Verification items for the finished model (mm, model axes). A direction names the side the tool comes from. Coordinates: 2 decimals unless noted, no trailing zeros. Write each loop counter-clockwise with the first axis right and the second up, starting at its lowest first coordinate (ties: lowest second). Pieces come first, ordered by that corner, then holes. Notation, with made-up numbers: M 79,73 L 110,73 A21 ccw 110,81 Z; hole C 29.5,68.5 d8. An arc over 180 degrees is marked long. Answer in a Markdown table with one row per item.
from build123d import *

# Parameters (mm, degrees)
F1_DEPTH = 88.9


with BuildPart() as f1:
    # F0 (on Front) → F1 (new body)
    with BuildSketch(Plane.XZ):
        Polygon((53.412888, 0), (0, 167.077348), (-5.068147, 167.077348), (-64.475396, 4.895769), (-73.939636, 8.340181), (-71.767969, 14.307288), (-75.421233, 15.636856), (-77.5929, 9.669749), (-79.330342, 4.895769), (-79.330342, 0), (-66.222783, 0.125408), (-61.154637, 0.125408), (-41.877323, 52.752407), (-2.916649, 52.752407), (31.086335, 52.752407), (48.650388, 0), align=None)
        Polygon((29.563813, 57.514907), (-2.916649, 57.514907), (-40.132815, 57.514907), (-2.916649, 159.114907), align=None, mode=Mode.SUBTRACT)
    extrude(amount=F1_DEPTH)


solid = f1.part
1) Thickness scan on L1, parallel to X at y = -52, z = 67; L2, parallel to X at y = -20, z = 153.5; L3, parallel to X at y = -71.5, z = 57. Record the ranges inside material, lowest first. Write a range as [from, to].
Response values:
| item | result |
|---|---|
| L1 | x = [-41.73, -36.66], [26.53, 31.99] |
| L2 | x = [-10.04, -4.97], [-1.12, 4.34] |
| L3 | x = [-45.39, 35.19] |
2) Depth check by flat-ended pin: pin 1 (2 mm diameter, centred on y = -33.5, z = 40.5, fed in from +X); pin 2 (5 mm diameter, centred on x = -28.5, y = -16.5, fed in from -Z); pin 3 (3 mm diameter, centred on x = -13.5, z = 60.5, fed in from -Y); pin 4 (5.5 mm diameter, centred on x = -63, y = -25, fed in from -Z). Enter the tip coordinate at first touch or a pass-through.
Response values:
| item | result |
|---|---|
| pin 1 | stops at x = 40.79 |
| pin 2 | stops at z = 52.75 |
| pin 3 | passes through |
| pin 4 | stops at z = 0.13 |
3) Sectioned sample at B-B (x = 11.5). Record the cut outline in (y, z), then the cut area to 3 significant figures.
Response values:
| item | result |
|---|---|
| outline | M -88.9,52.75 L 0,52.75 L 0,57.51 L -88.9,57.51 Z; M -88.9,114.02 L 0,114.02 L 0,131.1 L -88.9,131.1 Z |
| area | 1,940 mm² |
4) Sectioned sample at A-A (y = -29.5). Record the cut outline in (x, z), then the cut area to 3 significant figures.
Response values:
| item | result |
|---|---|
| outline | M -79.33,0 L -66.22,0.13 L -61.15,0.13 L -41.88,52.75 L 31.09,52.75 L 48.65,0 L 53.41,0 L 0,167.08 L -5.07,167.08 L -64.48,4.9 L -73.94,8.34 L -71.77,14.31 L -75.42,15.64 L -77.59,9.67 L -79.33,4.9 Z; hole M -40.13,57.51 L 29.56,57.51 L -2.92,159.11 Z |
| area | 2,190 mm² |
5) Sectioned sample at C-C (z = 39.5). Record the cut outline in (x, y).
Response values:
| item | result |
|---|---|
| outline | M -51.8,-88.9 L -46.73,-88.9 L -46.73,0 L -51.8,0 Z; M 35.5,-88.9 L 40.79,-88.9 L 40.79,0 L 35.5,0 Z |
6) Tool access check on faces 1 (the face through (-51.65, -43.83, 26.07)), 2 (the face through (-73.569, -43.828, 14.963)), 3 (the face through (-21.785, -43.828, 107.604)). Record the directions out of +Z, -Z, +X, -X, +Y, -Y that give a thin tool (end or side, any length) a straight path to the whole face; none if there is none.
Response values:
| item | result |
|---|---|
| face 1 | -Z, +Y, -Y |
| face 2 | +Z, +Y, -Y |
| face 3 | +Y, -Y |
